from build123d import *

# Parameters (mm, degrees)
SKETCH1_R           = 20
BOSS_EXTRUDE1_DEPTH = 58
SKETCH7_R           = 2.5
BOSS_EXTRUDE2_DEPTH = 25
SKETCH8_W           = 50
SKETCH8_H           = 10
BOSS_EXTRUDE3_DEPTH = 2
SKETCH9_W           = 3
SKETCH9_H           = 10
BOSS_EXTRUDE4_DEPTH = 20
SKETCH10_W          = 3
SKETCH10_H          = 10
BOSS_EXTRUDE5_DEPTH = 20


with BuildPart() as part:
    # Sketch1 → Boss-Extrude1 (new body)
    with BuildSketch(Plane.XY):
        Circle(SKETCH1_R)
    extrude(amount=BOSS_EXTRUDE1_DEPTH)

    # Sketch7 → Boss-Extrude2 (add)
    with BuildSketch(Plane(origin=(0, 0, 0), x_dir=(1, 0, 0), z_dir=(0, 1, 0))):
        with Locations((0, -3.561686207)):
            Circle(SKETCH7_R)
    boss_extrude2 = extrude(amount=BOSS_EXTRUDE2_DEPTH)

    # Sketch8 → Boss-Extrude3 (add)
    with BuildSketch(Plane.XY.offset(58)):
        Rectangle(SKETCH8_W, SKETCH8_H)
    extrude(amount=BOSS_EXTRUDE3_DEPTH)

    # Sketch9 → Boss-Extrude4 (add)
    with BuildSketch(Plane.XY.offset(60)):
        with Locations((-23.5, 0)):
            Rectangle(SKETCH9_W, SKETCH9_H)
    extrude(amount=BOSS_EXTRUDE4_DEPTH)

    # Sketch10 → Boss-Extrude5 (add)
    with BuildSketch(Plane.XY.offset(60)):
        with Locations((23.5, 0)):
            Rectangle(SKETCH10_W, SKETCH10_H)
    extrude(amount=BOSS_EXTRUDE5_DEPTH)

    # Mirror1: Boss-Extrude2 across plane
    add(boss_extrude2.mirror(Plane.ZX))


solid = part.part
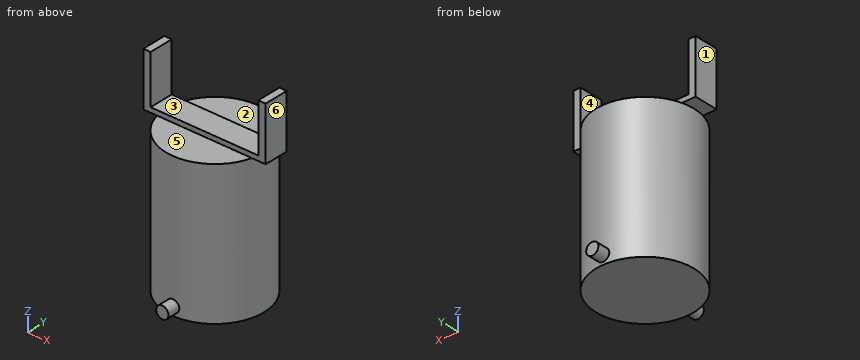
Can you work these out from the model? Positions are in its coordinate system, mm. Face numbers are marked on the shaded views. A direction names the side the tool comes from. Round coordinates to 2 decimals unless told otherwise and drop trailing zeros. Write each loop counter-clockwise with the first axis right and the second up, starting at its lowest first coordinate (ties: lowest second). Pieces come first, ordered by that corner, then holes. Notation, with made-up numbers: M 29,49 L 47,49 A11 ccw 47,61 Z; hole C -16,-31.75 d1. An arc over 180 degrees is marked long. Use a Markdown table: item, result.
Item 1: We'd pull the mould along X, two halves only. Please class the marked faces 4, 5 and 6: released by +X, released by -X, zero draft, split by the parting line, or undercut.
Found:
| item | result |
|---|---|
| face 4 | undercut |
| face 5 | zero draft |
| face 6 | released by +X |
Item 2: If I drill on line 1 along X through (y, z) = (-4, 65); line 2 along Z through (x, y) = (-12.5, 14); line 3 along Y through (x, z) = (7.5, 59.5), over which ranges is the centre line in solid material (lowest first)? Write a range as [from, to].
Found:
| item | result |
|---|---|
| line 1 | x = [-25, -22], [22, 25] |
| line 2 | z = [0, 58] |
| line 3 | y = [-5, 5] |
Item 3: I want a section at D-D (x = 0). List the corners of the cut face in (y, z) for me, and give its area (3 significant figures).
Found:
| item | result |
|---|---|
| outline | M -25,1.06 L -20,1.06 L -20,0 L 20,0 L 20,1.06 L 25,1.06 L 25,6.06 L 20,6.06 L 20,58 L 5,58 L 5,60 L -5,60 L -5,58 L -20,58 L -20,6.06 L -25,6.06 Z |
| area | 2,390 mm2 |
Item 4: I want a section at A-A (z = 69.5). List the corners of the cut face in (x, y) for me, and give its area (3 significant figures).
Found:
| item | result |
|---|---|
| outline | M -25,-5 L -22,-5 L -22,5 L -25,5 Z; M 22,-5 L 25,-5 L 25,5 L 22,5 Z |
| area | 60.0 mm2 |
Item 5: For pin 1 Ø12 at (x, y) = (-2.5, 12.5) entering from +Z; pin 2 Ø17.5 at (x, z) = (-3, 72.5) entering from -Y; pin 3 Ø6 at (y, z) = (-5.5, 44.5) entering from +X; pin 4 Ø4 at (y, z) = (-19.5, 38) entering from +X, each with a flat end and sliding along its axis, tell me the tip position at first contact or that it passes through.
Found:
| item | result |
|---|---|
| pin 1 | stops at z = 58 |
| pin 2 | passes through |
| pin 3 | stops at x = 19.84 |
| pin 4 | stops at x = 9.68 |
Item 6: I want a section at C-C (y = 0). List the corners of the cut face in (x, z) for me, and give its area (3 significant figures).
Found:
| item | result |
|---|---|
| outline | M -25,58 L -20,58 L -20,0 L 20,0 L 20,58 L 25,58 L 25,80 L 22,80 L 22,60 L -22,60 L -22,80 L -25,80 Z |
| area | 2,540 mm2 |
Item 7: I want a section at B-B (x = -16). List the corners of the cut face in (y, z) for me, and give its area (3 significant figures).
Found:
| item | result |
|---|---|
| outline | M -12,0 L 12,0 L 12,58 L 5,58 L 5,60 L -5,60 L -5,58 L -12,58 Z |
| area | 1,410 mm2 |
Item 8: Which directions (+Z, -Z, +X, -X, +Y, -Y) give clear straight access to the entire face, cutting with the end or side of a thin tool? Please do the marked faces 1, 2 and 3.
Found:
| item | result |
|---|---|
| face 1 | +Z, -Z, -X, +Y, -Y |
| face 2 | +Z, +X, -X, +Y |
| face 3 | +Z, +Y, -Y |
